```python
from build123d import *

# Parameters (mm, degrees)
SKETCH5_R               = 12.721239978
CUT_EXTRUDE1_DEPTH      = 1100
CUT_EXTRUDE1_DEPTH_BACK = 1100
SKETCH4_4_W             = 45.098856354
SKETCH4_4_H             = 1.822787056
SKETCH4_4_W_2           = 44.950171806
SKETCH4_4_H_2           = 4.046424606
SKETCH4_4_W_3           = 45.020896592
SKETCH4_4_H_3           = 3.001393106
CUT_EXTRUDE2_DEPTH      = 21
CUT_EXTRUDE2_DEPTH_BACK = 21


with BuildPart() as part:
    # Sketch4 → Revolve-Thin1 (revolve)
    with BuildSketch(Plane.XY):
        Polygon((-243.719110407, 0), (-243.719110407, 15), (-46.219110407, 15), (-46.219110407, 20), (-21.219110407, 20), (-18.010973852, 15), (630.572753038, 15), (633.780889593, 20), (658.780889593, 20), (658.780889593, 15), (856.280889593, 15), (856.280889593, 0), (846.280889593, 0), (846.280889593, 5), (648.780889593, 5), (648.780889593, 10), (639.246054132, 10), (636.037917577, 5), (-23.476138391, 5), (-26.684274946, 10), (-36.219110407, 10), (-36.219110407, 5), (-233.719110407, 5), (-233.719110407, 0), align=None)
    revolve(axis=Axis((-243.719110407, 0, 0), (1, 0, 0)))

    # Sketch5 → Cut-Extrude1 (cut, two sides)
    with BuildSketch(Plane.ZY.offset(243.719110407)) as cut_extrude1_sk:
        Circle(SKETCH5_R)
    extrude(amount=CUT_EXTRUDE1_DEPTH, mode=Mode.SUBTRACT)
    extrude(cut_extrude1_sk.sketch, amount=-CUT_EXTRUDE1_DEPTH_BACK, mode=Mode.SUBTRACT)

    # Sketch4_4 → Cut-Extrude2 (cut, two sides)
    with BuildSketch(Plane.XY) as cut_extrude2_sk:
        with Locations((-180.719110407, 0)):
            Rectangle(SKETCH4_4_W, SKETCH4_4_H)
        with Locations((118.780889593, 0)):
            Rectangle(SKETCH4_4_W_2, SKETCH4_4_H_2)
        with Locations((493.780889593, 0)):
            Rectangle(SKETCH4_4_W_3, SKETCH4_4_H_3)
        with Locations((793.280889593, 0)):
            Rectangle(SKETCH4_4_W_3, SKETCH4_4_H_3)
    extrude(amount=CUT_EXTRUDE2_DEPTH, mode=Mode.SUBTRACT)
    extrude(cut_extrude2_sk.sketch, amount=-CUT_EXTRUDE2_DEPTH_BACK, mode=Mode.SUBTRACT)


solid = part.part
```
The listing builds one solid part. Answer for the finished solid, in the listing's coordinates (mm). A direction names the side the tool comes from. Give positions to 0.01 mm unless a question says otherwise; leave off trailing zeros. Order: outer loops, then holes, each group sorted by start corner. A loop starts at its lowest first (then second) coordinate and runs counter-clockwise, first axis right, second up. Notation, with made-up numbers: (32.5, 9) - (88.5, 9) arc R32 cw to (88.5, 48) - close; hole circle Ø11 at (33, 21). An arc over 180 degrees is marked (long way). Use one line per item in the form item = value. Start each with the question number.
(1) The mould has two halves that part along Y. Classify faces 1 (the cylindrical face through (298.58, -4.87, 11.75)), 2 (the conical face through (-18.17, 14.54, 4.58)), 3 (the flat face through (856.281, -7, -11)): released by +Y, released by -Y, zero draft, split by the parting line, or undercut.
(2) A cutting plane is placed at A-A, the plane z = 0. Write down the section's boundary in (x, y).
(3) Flat-ended cylindrical pins translate along their axes: pin 1 Ø1.8 at (x, z) = (782.5, 14) entering from +Y; pin 2 Ø1.1 at (x, z) = (488.5, 13.5) entering from +Y; pin 3 Ø5 at (x, z) = (703.5, 15.5) entering from -Y. Find the tip coordinate at first contact, or state that the pin passes through.
(4) A cutting plane is placed at B-B, the plane x = 619. Write down the section's boundary in (y, z).
(5) Consider line 1 (Z direction, x = 195, y = 0); line 2 (Y direction, x = -157.5, z = 2.5); line 3 (X direction, y = 8, z = -18). Determine where each line is inside the solid, lowest interval first. Write a range as from..to.
(6) For faces 4 (the flat face through (-46.219, -3, 15)), 5 (the cylindrical face through (310.821, -14.985, 0.66)), 6 (the flat face through (658.781, 3, 15)), determine the directions among +Z, -Z, +X, -X, +Y, -Y from which every point of the face is accessible in a straight line to the end or side of a thin tool.
Ans:
q1.face_1 = undercut
q1.face_2 = split by the parting line
q1.face_3 = zero draft
q2.outline = (-243.72, -15) - (-46.22, -15) - (-46.22, -20) - (-21.22, -20) - (-18.01, -15) - (630.57, -15) - (633.78, -20) - (658.78, -20) - (658.78, -15) - (856.28, -15) - (856.28, -12.72) - (-243.72, -12.72) - close; (-243.72, 12.72) - (856.28, 12.72) - (856.28, 15) - (658.78, 15) - (658.78, 20) - (633.78, 20) - (630.57, 15) - (-18.01, 15) - (-21.22, 20) - (-46.22, 20) - (-46.22, 15) - (-243.72, 15) - close
q3.pin_1 = 7.31
q3.pin_2 = 7.57
q3.pin_3 = -7.48
q4.outline = circle Ø30 at (0, 0); hole circle Ø25.44 at (0, 0)
q5.line_1 = -15..-12.72, 12.72..15
q5.line_2 = -14.79..-12.47, 12.47..14.79
q5.line_3 = -46.22..-21.03, 633.59..658.78
q6.face_4 = -X
q6.face_5 = none
q6.face_6 = +X
